```python
from build123d import *

# Parameters (mm, degrees)
SKETCH2_W               = 286.300000032
SKETCH2_H               = 238.275
BOSS_EXTRUDE1_DEPTH     = 1.5875
SKETCH4_W               = 3.175
SKETCH4_H               = 38.1
SKETCH4_W_2             = 38.1
SKETCH4_H_2             = 6.35
WELD_TABS_EXTRUDE_DEPTH = 3.175
SKETCH5_R               = 1.5875
CUT_EXTRUDE1_DEPTH      = 3.175


with BuildPart() as part:
    # Sketch2 → Boss-Extrude1 (new body, symmetric)
    with BuildSketch(Plane.XY):
        with Locations((-144.737500016, 122.3125)):
            Rectangle(SKETCH2_W, SKETCH2_H)
    extrude(amount=BOSS_EXTRUDE1_DEPTH, both=True)

    # Sketch4 → Weld Tabs Extrude (add)
    with BuildSketch(Plane(origin=(0, 0, -1.5875), x_dir=(-1, 0, 0), z_dir=(0, 0, -1))):
        with Locations((0, 181.88125)):
            Rectangle(SKETCH4_W, SKETCH4_H)
        with Locations((0, 122.3125)):
            Rectangle(SKETCH4_W, SKETCH4_H)
        with Locations((0, 62.74375)):
            Rectangle(SKETCH4_W, SKETCH4_H)
        with Locations((72.368750008, 0)):
            Rectangle(SKETCH4_W_2, SKETCH4_H_2)
        with Locations((144.737500016, 0)):
            Rectangle(SKETCH4_W_2, SKETCH4_H_2)
        with Locations((217.106250024, 0)):
            Rectangle(SKETCH4_W_2, SKETCH4_H_2)
        with Locations((289.475000032, 181.88125)):
            Rectangle(SKETCH4_W, SKETCH4_H)
        with Locations((289.475000032, 122.3125)):
            Rectangle(SKETCH4_W, SKETCH4_H)
        with Locations((289.475000032, 62.74375)):
            Rectangle(SKETCH4_W, SKETCH4_H)
    extrude(amount=-WELD_TABS_EXTRUDE_DEPTH)

    # Sketch5 → Cut-Extrude1 (cut)
    with BuildSketch(Plane.XY.offset(1.5875)):
        with Locations((-0.464967985, 202.053782015)):
            Circle(SKETCH5_R)
        with Locations((-0.464967985, 142.485032015)):
            Circle(SKETCH5_R)
        with Locations((-0.464967985, 82.916282015)):
            Circle(SKETCH5_R)
        with Locations((-0.464967985, 161.708717985)):
            Circle(SKETCH5_R)
        with Locations((-0.464967985, 102.139967985)):
            Circle(SKETCH5_R)
        with Locations((-0.464967985, 42.571217985)):
            Circle(SKETCH5_R)
        with Locations((-289.010032047, 42.571217985)):
            Circle(SKETCH5_R)
        with Locations((-289.010032047, 82.916282015)):
            Circle(SKETCH5_R)
        with Locations((-289.010032047, 102.139967985)):
            Circle(SKETCH5_R)
        with Locations((-289.010032047, 142.485032015)):
            Circle(SKETCH5_R)
        with Locations((-289.010032047, 161.708717985)):
            Circle(SKETCH5_R)
        with Locations((-289.010032047, 202.053782015)):
            Circle(SKETCH5_R)
        with Locations((-52.196217993, 2.052467985)):
            Circle(SKETCH5_R)
        with Locations((-92.541282023, 2.052467985)):
            Circle(SKETCH5_R)
        with Locations((-124.564968001, 2.052467985)):
            Circle(SKETCH5_R)
        with Locations((-237.278782039, 2.052467985)):
            Circle(SKETCH5_R)
        with Locations((-196.933718009, 2.052467985)):
            Circle(SKETCH5_R)
        with Locations((-164.910032031, 2.052467985)):
            Circle(SKETCH5_R)
    extrude(amount=-CUT_EXTRUDE1_DEPTH, mode=Mode.SUBTRACT)


solid = part.part
```
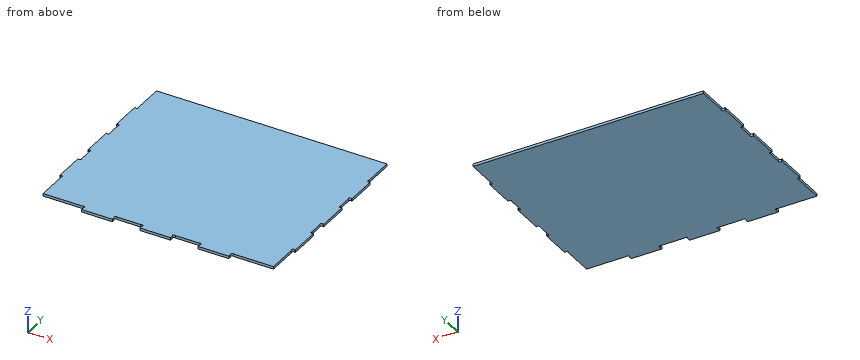
Geometry: final body of the model. Coordinates: model frame, mm. Coordinates: 2 decimals unless noted, no trailing zeros. Order: outer loops, then holes, each group sorted by start corner. A loop starts at its lowest first (then second) coordinate and runs counter-clockwise, first axis right, second up. Notation, with made-up numbers: (-6, 61) - (34, 61) arc R27 cw to (34, 78) - close; hole circle Ø9 at (53, 21). An arc over 180 degrees is marked (long way). Write each question's results on one line, items separated by ' | '.
1) Section A-A, the plane y = 217. Return loops of the section in (x, z), plus the area to 3 significant figures.
Results list:
outline: (-287.89, -1.59) - (-1.59, -1.59) - (-1.59, 1.59) - (-287.89, 1.59) - close | area: 909 mm^2
2) Line query: line 1 (Y direction, x = -39.5, z = 0.95) (3 decimals); line 2 (X direction, y = 19, z = -0.3); line 3 (X direction, y = 201.5, z = -1.3). Output: solid intervals per line, ascending. Write a range as from..to.
Results list:
line 1: 3.175..241.45 | line 2: -287.89..-1.59 | line 3: -287.52..-1.95
3) Pin query (flat end, axial travel): pin 1 (1.6 mm diameter, centred on y = -1, z = 0, fed in from +X); pin 2 (1.6 mm diameter, centred on y = 88.5, z = 0.5, fed in from +X); pin 3 (1 mm diameter, centred on y = 96, z = 0.5, fed in from -X). Return the tip coordinate at first contact, or that it passes through.
Results list:
pin 1: x = -53.32 | pin 2: x = -1.59 | pin 3: x = -287.89
